CAD build for the part. Positions are in the model's coordinates, mm. A direction names the side the tool comes from. Give positions to 0.01 mm unless a question says otherwise; leave off trailing zeros. Order: outer loops, then holes, each group sorted by start corner. A loop starts at its lowest first (then second) coordinate and runs counter-clockwise, first axis right, second up. Notation, with made-up numbers: M 6.5,53.25 L 32.5,53.25 A24 ccw 32.5,80.25 Z; hole C 19,-16.5 d11. An arc over 180 degrees is marked long. Put each result on its own line as item: value. Start each with the question number.
1) Cut at C-C (z = -32). Write the cut outline in (x, y) (3 decimals), and give its area (3 significant figures).
2) Cut at D-D (x = 10). Write the cut outline in (y, z), and give its area (3 significant figures).
3) Pin check, flat tips, straight feed: pin 1 (3 mm diameter, centred on x = 33.5, y = -12, fed in from +Z); pin 2 (1 mm diameter, centred on y = -10.5, z = -37.5, fed in from +X); pin 3 (8 mm diameter, centred on y = -6, z = -16, fed in from +X). Stop position of each tip, or through.
4) Tool access for faces 1 (the face through (45, 0, 0)), 2 (the face through (40.03, 26.96, -20.08)), 3 (the face through (24.605, 26.96, -37.373)): list every direction of +Z, -Z, +X, -X, +Y, -Y with a clear straight run to the whole face (end or side of a thin tool).
5) Drill centre lines: line 1 (Y direction, x = 16, z = -40.5); line 2 (X direction, y = -13.5, z = -34.5); line 3 (X direction, y = 25, z = -38.5). Where is each one in solid material? Low to high. Write a range as [from, to].
6) Cut at B-B (x = 40.5). Write the cut outline in (y, z) (3 decimals).
7) Cut at A-A (y = -9). Write the cut outline in (x, z) (3 decimals).
```python
from build123d import *

# Parameters (mm, degrees)
BOSS_EXTRUDE1_DEPTH = 25.3500001
BOSS_EXTRUDE2_START = 3.175
BOSS_EXTRUDE2_DEPTH = 3.175


with BuildPart() as part:
    # Sketch1 → Boss-Extrude1 (new, symmetric)
    with BuildSketch(Plane(origin=(0, 0, 0), x_dir=(1, 0, 0), z_dir=(0, 1, 0))):
        with BuildLine():
            Line((6.278041701, 42.721172648), (6.739662414, 45.862435342))
            ThreePointArc((6.739662414, 45.862435342), (35.079930703, 30.30155915), (46.355, 0))
            Line((46.355, 0), (43.18, 0))
            ThreePointArc((43.18, 0), (32.677195723, 28.226109893), (6.278041701, 42.721172648))
        make_face()
    extrude(amount=BOSS_EXTRUDE1_DEPTH, both=True)

    # Sketch4 → Boss-Extrude2 (add)
    with BuildSketch(Plane(origin=(0, 25.3500001, 0), x_dir=(1, 0, 0), z_dir=(0, 1, 0)).offset(BOSS_EXTRUDE2_START)):
        with BuildLine():
            Line((41.434019217, 20.784803982), (38.596072695, 19.361187271))
            ThreePointArc((38.596072695, 19.361187271), (32.269899408, 28.690869492), (23.744585805, 36.065316371))
            Line((23.744585805, 36.065316371), (25.490511231, 38.717177869))
            ThreePointArc((25.490511231, 38.717177869), (34.642686129, 30.800492249), (41.434019217, 20.784803982))
        make_face()
    extrude(amount=-BOSS_EXTRUDE2_DEPTH)


solid = part.part
```
Solution:
1. outline: M 28.992,-25.35 L 33.538,-25.35 L 33.538,28.525 L 28.992,28.525 Z
1. area: 245 mm²
2. outline: M -25.35,-45.26 L 25.35,-45.26 L 25.35,-42.01 L -25.35,-42.01 Z
2. area: 165 mm²
3. pin 1: z = -25.29
3. pin 2: x = 27.92
3. pin 3: x = 44.77
4. face 1: +Z, +X, -X, +Y, -Y
4. face 2: +Z, +X, +Y
4. face 3: -Z, -X, +Y
5. line 1: [-25.35, 25.35]
5. line 2: [25.97, 30.96]
5. line 3: [19.55, 25.82]
6. outline: M -25.35,-22.551 L 28.525,-22.551 L 28.525,-20.316 L 25.35,-20.316 L 25.35,-14.975 L -25.35,-14.975 Z
7. outline: M 6.278,-42.721 L 6.74,-45.862 A46.355 ccw 46.355,0 L 43.18,0 A43.18 cw Z
